```python
from build123d import *

# Parameters (mm, degrees)
ESBO_O1_R                = 9.05
ESBO_O1_R_2              = 3.5
RESSALTO_EXTRUS_O1_DEPTH = 1
FILETE1_R                = 0.3


with BuildPart() as part:
    # Esboço1 → Ressalto-extrusão1 (new body)
    with BuildSketch(Plane.XY):
        Circle(ESBO_O1_R)
        Circle(ESBO_O1_R_2, mode=Mode.SUBTRACT)
    extrude(amount=RESSALTO_EXTRUS_O1_DEPTH)

    # Filete1
    filete1_edges = [part.edges().sort_by_distance(p)[0] for p in [
        (-9.05, 0, 0),
        (-9.05, 0, 1),
        (-3.5, 0, 0),
        (-3.5, 0, 1),
    ]]
    fillet(filete1_edges, radius=FILETE1_R)


solid = part.part
```
Input: part model. Units: mm. Frame: model coordinates. Coordinates: 2 decimals unless noted, no trailing zeros. Write each loop counter-clockwise with the first axis right and the second up, starting at its lowest first coordinate (ties: lowest second). Pieces come first, ordered by that corner, then holes.
1) Section C-C on z = 0.5. Output: boundary loops of the cut face in (x, y), and give its area (3 significant figures).
2) Section A-A on x = 0. Output: boundary loops of the cut face in (y, z), and give its area (3 significant figures).
3) Pin query (flat end, axial travel): pin 1 Ø10 at (x, y) = (5, 7) entering from -Z. Return the tip coordinate at first contact, or that it passes through.
4) Mould query, pull axis X, two halves, no side actions, for faces 1 (the flat face through (2, -4, 1)), 2 (the cylindrical face through (8.63, 2.72, 0.5)), 3 (the cylindrical face through (3.233, -1.341, 0.497)). Classes: pulls with the +X half, pulls with the -X half, needs draft (parallel to the pull), parting line crosses it, or undercut.
5) Material intervals for line 1 along Y through (x, z) = (0, 0.45); line 2 along Y through (x, z) = (3, 0.55); line 3 along X through (y, z) = (-2, 0.15), sorted ascending.
Check result:
1. outline: circle Ø18.1 at (0, 0); hole circle Ø7 at (0, 0)
1. area: 219 mm2
2. outline: (-9.05, 0.3) arc R0.3 ccw to (-8.75, 0) - (-3.8, 0) arc R0.3 ccw to (-3.5, 0.3) - (-3.5, 0.7) arc R0.3 ccw to (-3.8, 1) - (-8.75, 1) arc R0.3 ccw to (-9.05, 0.7) - close; (3.5, 0.3) arc R0.3 ccw to (3.8, 0) - (8.75, 0) arc R0.3 ccw to (9.05, 0.3) - (9.05, 0.7) arc R0.3 ccw to (8.75, 1) - (3.8, 1) arc R0.3 ccw to (3.5, 0.7) - close
2. area: 10.9 mm2
3. pin 1: stops at z = 0
4. face 1: needs draft
4. face 2: parting line crosses it
4. face 3: undercut
5. line 1: y = -9.05 to -3.5, 3.5 to 9.05
5. line 2: y = -8.54 to -1.8, 1.8 to 8.54
5. line 3: x = -8.79 to -2.92, 2.92 to 8.79
